Source: CAD feature listing. Evaluate the final solid. Frame: model axes, mm. Round coordinates to 2 decimals unless told otherwise and drop trailing zeros. Write each loop counter-clockwise with the first axis right and the second up, starting at its lowest first coordinate (ties: lowest second). Pieces come first, ordered by that corner, then holes. Notation, with made-up numbers: M 88,-37.75 L 111,-37.75 A20 ccw 111,-22.75 Z; hole C 0.25,63.5 d11. An arc over 180 degrees is marked long. Answer in a Markdown table with one row per item. Add a question column.
Item 1: Material intervals for probe 1 along Z at (x, y) = (15.5, 27.75); probe 2 along Z at (x, y) = (31, 27.15); probe 3 along X at (y, z) = (27.45, 63), sorted ascending.
Item 2: Cut plane A-A on y = 27.8. Return loops of the section in (x, z).
Item 3: Cut plane B-B on x = 76.5. Return loops of the section in (y, z).
from build123d import *

# Parameters (mm, degrees)
BOSS_EXTRUDE1_DEPTH   = 327.5
BOSS_EXTRUDE1_2_DEPTH = 327.5
BOSS_EXTRUDE2_DEPTH   = 2
BOSS_EXTRUDE4_DEPTH   = 1
SKETCH4_W             = 100
SKETCH4_H             = 8.5
BOSS_EXTRUDE5_DEPTH   = 2
BOSS_EXTRUDE6_DEPTH   = 1
SKETCH7_R             = 5
SKETCH7_W             = 96
SKETCH7_H             = 1
CUT_EXTRUDE2_DEPTH    = 1
SKETCH8_W             = 100
SKETCH8_H             = 13.5
CUT_EXTRUDE3_DEPTH    = 400
SKETCH9_W             = 1
SKETCH9_H             = 5
CUT_EXTRUDE4_DEPTH    = 84.5
SKETCH10_W            = 83
SKETCH10_H            = 228.97918472
BOSS_EXTRUDE7_DEPTH   = 1
SKETCH12_W            = 120.619846079
SKETCH12_H            = 19.843524077
CUT_EXTRUDE6_DEPTH    = 400


with BuildPart() as part:
    # Sketch1 → Boss-Extrude1 (new body)
    with BuildSketch(Plane.XY):
        Polygon((0, 0), (0, 8.5), (1, 8.5), (1, 13.5), (2, 13.5), (2, 2), (13.5, 2), (13.5, 1), (8.5, 1), (8.5, 0), align=None)
    extrude(amount=BOSS_EXTRUDE1_DEPTH)



with BuildPart() as body_2:
    # Sketch1 → Boss-Extrude1 2 (new body)
    with BuildSketch(Plane.XY):
        Polygon((100, 0), (91.5, 0), (91.5, 1), (86.5, 1), (86.5, 2), (98, 2), (98, 13.5), (99, 13.5), (99, 8.5), (100, 8.5), align=None)
    extrude(amount=BOSS_EXTRUDE1_2_DEPTH)


with BuildPart() as part_1:
    add(part.part)

    add(body_2.part)  # Boss-Extrude2 merges body 2
    # Sketch2 → Boss-Extrude2 (add)
    with BuildSketch(Plane(origin=(0, 2, 0), x_dir=(1, 0, 0), z_dir=(0, 1, 0))):
        Polygon((86.5, 0), (13.5, -73), (13.5, -85.02081528), (86.5, -12.02081528), align=None)
    extrude(amount=-BOSS_EXTRUDE2_DEPTH)

    # Sketch3 → Boss-Extrude4 (add)
    with BuildSketch(Plane.XZ.offset(-1)):
        Polygon((13.5, 73), (13.5, 85.02081528), (8.5, 90.02081528), (8.5, 78), align=None)
        Polygon((86.5, 0), (86.5, 12.02081528), (91.5, 7.02081528), (91.5, 0), align=None)
    extrude(amount=BOSS_EXTRUDE4_DEPTH)

    # Sketch4 → Boss-Extrude5 (add)
    with BuildSketch(Plane.XZ):
        with Locations((50, 323.25)):
            Rectangle(SKETCH4_W, SKETCH4_H)
    extrude(amount=-BOSS_EXTRUDE5_DEPTH)

    # Sketch7 → Cut-Extrude2 (cut)
    with BuildSketch(Plane(origin=(0, 2, 0), x_dir=(1, 0, 0), z_dir=(0, 1, 0))):
        with Locations((26.5, -326.5)):
            Circle(SKETCH7_R)
        with Locations((73.5, -326.5)):
            Circle(SKETCH7_R)
        with Locations((50, -327)):
            Rectangle(SKETCH7_W, SKETCH7_H)
    extrude(amount=-CUT_EXTRUDE2_DEPTH, mode=Mode.SUBTRACT)


with BuildPart() as body_2_2:
    # Sketch5 → Boss-Extrude6 (new body)
    with BuildSketch(Plane(origin=(0, 2, 0), x_dir=(1, 0, 0), z_dir=(0, 1, 0))):
        Polygon((13.5, -65.928932188), (79.428932188, 0), (86.5, 0), (13.5, -73), align=None)
    extrude(amount=-BOSS_EXTRUDE6_DEPTH)


with BuildPart() as body_3:
    # Mirror1: mirrored copy
    add(body_2_2.part.mirror(Plane(origin=(1, 13.5, 327.5), x_dir=(0, 0, 1), z_dir=(0, -1, 0))))


with BuildPart() as body_4:
    # Mirror1 2: mirrored copy
    add(part_1.part.mirror(Plane(origin=(1, 13.5, 327.5), x_dir=(0, 0, 1), z_dir=(0, -1, 0))))

    # Sketch9 → Cut-Extrude4 (cut)
    with BuildSketch(Plane(origin=(0, 0, 0), x_dir=(-1, 0, 0), z_dir=(0, 0, -1))):
        with Locations((-1.5, 16)):
            Rectangle(SKETCH9_W, SKETCH9_H)
    extrude(amount=-CUT_EXTRUDE4_DEPTH, mode=Mode.SUBTRACT)


with BuildPart() as cut_extrude3_tool:
    # Sketch8 → Cut-Extrude3 (new body)
    with BuildSketch(Plane(origin=(0, 0, 0), x_dir=(-1, 0, 0), z_dir=(0, 0, -1))):
        with Locations((-50, 6.75)):
            Rectangle(SKETCH8_W, SKETCH8_H)
    extrude(amount=-CUT_EXTRUDE3_DEPTH)


with BuildPart() as part_2:
    add(part_1.part)

    # Cut-Extrude3: cut by cut_extrude3_tool
    add(cut_extrude3_tool.part, mode=Mode.SUBTRACT)


with BuildPart() as body_2_2_1:
    add(body_2_2.part)

    # Cut-Extrude3: cut by cut_extrude3_tool
    add(cut_extrude3_tool.part, mode=Mode.SUBTRACT)


with BuildPart() as body_3_2:
    # Sketch10 → Boss-Extrude7 (new body)
    with BuildSketch(Plane(origin=(0, 27, 0), x_dir=(1, 0, 0), z_dir=(0, 1, 0))):
        Polygon((91.5, -7.02081528), (8.5, -90.02081528), (91.5, -90.02081528), align=None)
        with Locations((50, -204.51040764)):
            Rectangle(SKETCH10_W, SKETCH10_H)
    extrude(amount=BOSS_EXTRUDE7_DEPTH)


with BuildPart() as cut_extrude6_tool:
    # Sketch12 → Cut-Extrude6 (new body)
    with BuildSketch(Plane.XY.offset(327.5)):
        with Locations((60.30992304, 17.078237962)):
            Rectangle(SKETCH12_W, SKETCH12_H)
    extrude(amount=-CUT_EXTRUDE6_DEPTH)


with BuildPart() as body_3_1:
    add(body_3.part)

    # Cut-Extrude6: cut by cut_extrude6_tool
    add(cut_extrude6_tool.part, mode=Mode.SUBTRACT)


with BuildPart() as body_4_1:
    add(body_4.part)

    # Cut-Extrude6: cut by cut_extrude6_tool
    add(cut_extrude6_tool.part, mode=Mode.SUBTRACT)


solid = body_3_2.part
Results below:
| question | item | result |
|---|---|---|
| 1 | probe 1 | 83.02 to 319 |
| 1 | probe 2 | 67.52 to 319 |
| 1 | probe 3 | 35.52 to 91.5 |
| 2 | outline | M 8.5,90.02 L 91.5,7.02 L 91.5,319 L 8.5,319 Z |
| 3 | outline | M 27,22.02 L 28,22.02 L 28,319 L 27,319 Z |
